from build123d import *

# Parameters (mm, degrees)
MAIN_DEPTH                      = 20
ESQUISSE2_R                     = 1.6
TOPHOLE_DEPTH                   = 5
R_P_TITION_LIN_AIRE1_COUNT      = 4
R_P_TITION_LIN_AIRE1_PITCH      = 20
R_P_TITION_LIN_AIRE1_COUNT_DIR2 = 2
R_P_TITION_LIN_AIRE1_PITCH_DIR2 = 10


with BuildPart() as part:
    # Esquisse1 → Main (new body)
    with BuildSketch(Plane.XY):
        Polygon((-5, 0), (-5, 3), (-1.45, 3), (-1.45, 4), (1.45, 4), (1.45, 3), (5, 3), (5, 0), align=None)
    main = extrude(amount=MAIN_DEPTH)

    # Esquisse2 → TopHole (cut, through all)
    with BuildSketch(Plane(origin=(0, 4, 0), x_dir=(1, 0, 0), z_dir=(0, 1, 0))):
        with Locations((0, -5)):
            Circle(ESQUISSE2_R)
        with Locations((0, -15)):
            Circle(ESQUISSE2_R)
    tophole = extrude(amount=-TOPHOLE_DEPTH, mode=Mode.SUBTRACT)

    # Répétition linéaire1: Main, TopHole 4 × 2
    with Locations(*[(-j * R_P_TITION_LIN_AIRE1_PITCH_DIR2, 0, i * R_P_TITION_LIN_AIRE1_PITCH) for i in range(R_P_TITION_LIN_AIRE1_COUNT) for j in range(R_P_TITION_LIN_AIRE1_COUNT_DIR2) if (i, j) != (0, 0)]):
        add(main)
        add(tophole, mode=Mode.SUBTRACT)


solid = part.part
Read the model definition and answer for the solid it produces. Units are mm, in the model's axes. A direction names the side the tool comes from. Coordinates: 2 decimals unless noted, no trailing zeros. Loops run counter-clockwise (first coordinate to the right, second up) from the corner with the lowest first, then second, coordinate; pieces in that order, holes last. Notation, with made-up numbers: (-12.5, 64.25) -> (2.5, 64.25) arc R10 ccw to (2.5, 80.25) -> close; hole circle Ø9 at (47, 12). An arc over 180 degrees is marked (long way). Write item = value, one per line. Start each with the question number.
1) The part is cut by section C-C, the plane x = -5.5. Determine the outline of the cut face in (y, z), plus the area to 3 significant figures.
2) The mould has two halves that part along X. Classify faces 3 (the face through (-11.6, 2.03, 4.93)), 4 (the face through (0, 4, 20)), 5 (the face through (5, 2, 39)): pulls with the +X half, pulls with the -X half, needs draft (parallel to the pull), parting line crosses it, or undercut.
3) Given P1, Ø4, axis at x = 3.5, z = 46, coming from the +Y side; P2, Ø0.8, axis at y = 3.5, z = 78, coming from the +X side; P3, Ø0.8, axis at y = 3.5, z = 38.5, coming from the -X side, each flat-ended and moving along its own axis, determine where each tip first touches the part or whether it passes through.
4) The part is cut by section B-B, the plane x = 0. State how many separate pieces and enclosed holes the cut face has, plus the area to 3 significant figures.
5) The part is cut by section A-A, the plane z = 5. Determine the outline of the cut face in (x, y), plus the area to 3 significant figures.
6) Find the intervals of material crossed by L1, parallel to X at y = 2.8, z = 15; L2, parallel to X at y = 2.85, z = 64; L3, parallel to X at y = 3.65, z = 41.5, in increasing order. Write a range as from..to.
7) For faces 1 (the face through (-5, 2, 0)), 2 (the face through (-13, 3, 39)), determine the directions among +Z, -Z, +X, -X, +Y, -Y from which every point of the face is accessible in a straight line to the end or side of a thin tool.
Result:
q1.outline = (0, 0) -> (3, 0) -> (3, 80) -> (0, 80) -> close
q1.area = 240 mm²
q2.face_3 = undercut
q2.face_4 = needs draft
q2.face_5 = pulls with the +X half
q3.P1 = 3
q3.P2 = 1.45
q3.P3 = -11.45
q4.separate_pieces = 9
q4.enclosed_holes = 0
q4.area = 218 mm²
q5.outline = (-15, 0) -> (-11.6, 0) -> (-11.6, 3) -> (-15, 3) -> close; (-8.4, 0) -> (-1.6, 0) -> (-1.6, 3) -> (-8.4, 3) -> close; (1.6, 0) -> (5, 0) -> (5, 3) -> (1.6, 3) -> close
q5.area = 40.8 mm²
q6.L1 = -15..-11.6, -8.4..-1.6, 1.6..5
q6.L2 = -15..-11.25, -8.75..-1.25, 1.25..5
q6.L3 = -11.45..-8.55, -1.45..1.45
q7.face_1 = -Z, +X, -X, +Y, -Y
q7.face_2 = +Z, -Z, -X, +Y
